Geometry check sheet. Reference: drawing and pictorial views, mm from the part's lowest x, y, z. Round coordinates to 2 decimals unless told otherwise and drop trailing zeros. Write each loop counter-clockwise with the first axis right and the second up, starting at its lowest first coordinate (ties: lowest second). Pieces come first, ordered by that corner, then holes. Notation, with made-up numbers: (-25, 68) - (15, 68) arc R25 ccw to (15, 103) - close; hole circle Ø10 at (-27.75, 34). An arc over 180 degrees is marked (long way). Use one line per item in the form item = value. Start each with the question number.
1) Section check C-C (y = 18.5). Record the boundary of the cut face in (x, z) (1 decimal).
2) Gauge pin test, flat ends, axial feed: P1, Ø6, axis at x = 90.5, y = 42.5, coming from the +Z side; P2, Ø16, axis at x = 11, y = 11, coming from the +Z side; P3, Ø1.5, axis at y = 80, z = 5, coming from the -X side; P4, Ø1.5, axis at y = 23, z = 3, coming from the -X side. Record the tip position at first contact, or that the pin passes through.
3) Scan lines: probe 1 along X at (y, z) = (4.5, 3.7) (1 decimal); probe 2 along X at (y, z) = (9, 4.85) (1 decimal); probe 3 along X at (y, z) = (13, 4.45) (1 decimal). Record each from-to range of solid material in increasing order.
4) Section check B-B (z = 3). Count the separate pieces of the cut face and the enclosed holes in it, then the cut area to 3 significant figures.
5) Section check D-D (y = 35.25). Record the boundary of the cut face in (x, z) (1 decimal).
6) Draft check along X on the marked faces 1, 2 and 3. Enter one of: +X half, -X half, draft (parallel to the pull), parting line (faces both ways), or undercut.
7) Section check A-A (x = 92.5). Record the boundary of the cut face in (y, z) (1 decimal), then the cut area to 3 significant figures.
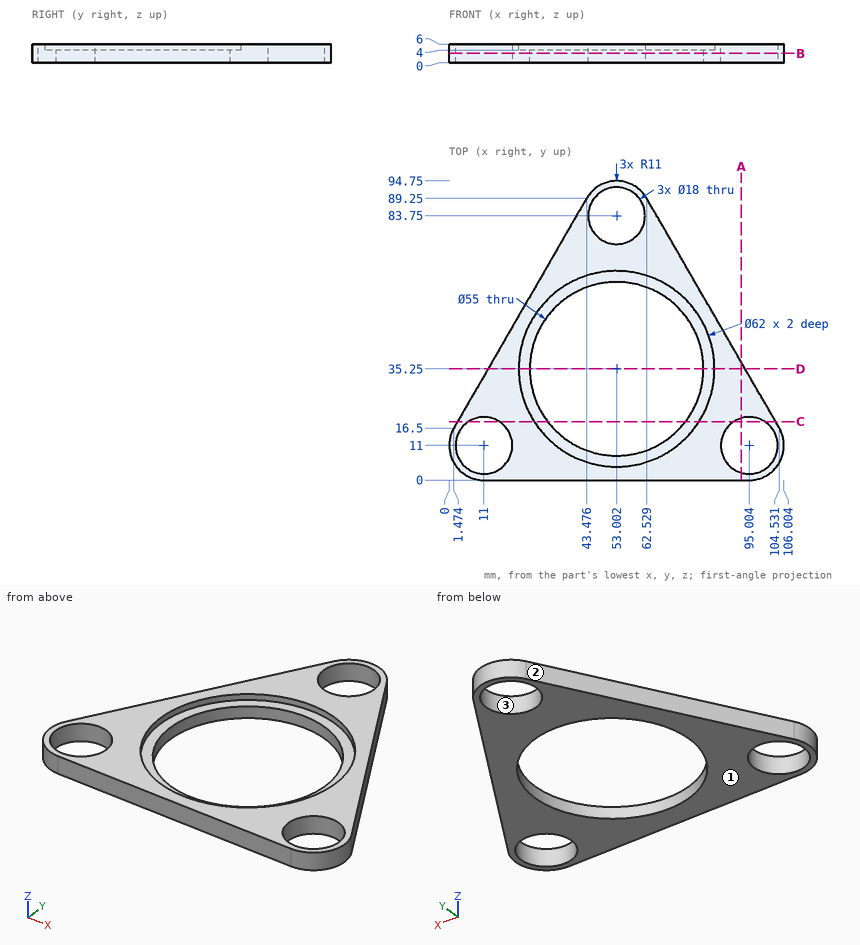
Results are:
q1.outline = (2.6, 0) - (6, 0) - (6, 6) - (2.6, 6) - close; (16, 0) - (31.2, 0) - (31.2, 4) - (26.9, 4) - (26.9, 6) - (16, 6) - close; (74.8, 0) - (90, 0) - (90, 6) - (79.1, 6) - (79.1, 4) - (74.8, 4) - close; (100, 0) - (103.4, 0) - (103.4, 6) - (100, 6) - close
q2.P1 = 6
q2.P2 = through
q2.P3 = 37.7
q2.P4 = 4.79
q3.probe_1 = 2.1 to 4.8, 17.2 to 88.8, 101.2 to 103.9
q3.probe_2 = 0.2 to 2.2, 19.8 to 36.5, 69.5 to 86.2, 103.8 to 105.8
q3.probe_3 = 0.2 to 2.2, 19.8 to 31.4, 74.6 to 86.2, 103.8 to 105.8
q4.separate_pieces = 1
q4.enclosed_holes = 4
q4.area = 3,070 mm²
q5.outline = (12.3, 0) - (25.5, 0) - (25.5, 4) - (22, 4) - (22, 6) - (12.3, 6) - close; (80.5, 0) - (93.7, 0) - (93.7, 6) - (84, 6) - (84, 4) - (80.5, 4) - close
q6.face_1 = draft
q6.face_2 = -X half
q6.face_3 = undercut
q7.outline = (0, 0) - (2.4, 0) - (2.4, 6) - (0, 6) - close; (19.6, 0) - (37.3, 0) - (37.3, 6) - (19.6, 6) - close
q7.area = 120 mm²
